Read the model definition and answer for the solid it produces. Units are mm, in the model's axes. A direction names the side the tool comes from. Round coordinates to 2 decimals unless told otherwise and drop trailing zeros. Order: outer loops, then holes, each group sorted by start corner. A loop starts at its lowest first (then second) coordinate and runs counter-clockwise, first axis right, second up. Notation, with made-up numbers: M 81.25,9 L 94.25,9 A14 ccw 94.25,24 Z; hole C -16,-12 d5. An arc over 180 degrees is marked long. Answer as CSV lines item,"result".
```python
from build123d import *

# Parameters (mm, degrees)
SALIENTE_EXTRUIR1_DEPTH = 5
REDONDEO1_R             = 30
CORTAR_EXTRUIR1_REACH   = 264.202
CROQUIS2_R              = 2


with BuildPart() as part:
    # Croquis1 → Saliente-Extruir1 (new body)
    with BuildSketch(Plane.XY):
        Polygon((-30, 0), (0, 0), (0, 5), (10, 5), (10, 215), (-150, 215), (-150, 170), (-120, 170), (-120, 175), (-40, 175), (-40, 5), (-30, 5), align=None)
    extrude(amount=SALIENTE_EXTRUIR1_DEPTH)

    # Redondeo1
    redondeo1_edges = [part.edges().sort_by_distance(p)[0] for p in [
        (-40, 175, 2.5),
        (-150, 215, 2.5),
        (10, 215, 2.5),
    ]]
    fillet(redondeo1_edges, radius=REDONDEO1_R)

    # Croquis2 → Cortar-Extruir1 (cut, up to next)
    with BuildSketch(Plane.XY.offset(5), mode=Mode.PRIVATE) as cortar_extruir1_sk1:
        with Locations((-7.5, 25)):
            Circle(CROQUIS2_R)
    cortar_extruir1_tool1 = extrude(cortar_extruir1_sk1.sketch, amount=-CORTAR_EXTRUIR1_REACH, mode=Mode.PRIVATE) & part.part
    # Croquis2 → Cortar-Extruir1 (cut, up to next)
    with BuildSketch(Plane.XY.offset(5), mode=Mode.PRIVATE) as cortar_extruir1_sk2:
        with Locations((-22.5, 25)):
            Circle(CROQUIS2_R)
    cortar_extruir1_tool2 = extrude(cortar_extruir1_sk2.sketch, amount=-CORTAR_EXTRUIR1_REACH, mode=Mode.PRIVATE) & part.part
    # Croquis2 → Cortar-Extruir1 (cut, up to next)
    with BuildSketch(Plane.XY.offset(5), mode=Mode.PRIVATE) as cortar_extruir1_sk3:
        with Locations((-127.5, 195)):
            Circle(CROQUIS2_R)
    cortar_extruir1_tool3 = extrude(cortar_extruir1_sk3.sketch, amount=-CORTAR_EXTRUIR1_REACH, mode=Mode.PRIVATE) & part.part
    # Croquis2 → Cortar-Extruir1 (cut, up to next)
    with BuildSketch(Plane.XY.offset(5), mode=Mode.PRIVATE) as cortar_extruir1_sk4:
        with Locations((-142.5, 195)):
            Circle(CROQUIS2_R)
    cortar_extruir1_tool4 = extrude(cortar_extruir1_sk4.sketch, amount=-CORTAR_EXTRUIR1_REACH, mode=Mode.PRIVATE) & part.part
    add(cortar_extruir1_tool1.solids().sort_by_distance((-7.5, 25, 5))[0], mode=Mode.SUBTRACT)
    add(cortar_extruir1_tool2.solids().sort_by_distance((-22.5, 25, 5))[0], mode=Mode.SUBTRACT)
    add(cortar_extruir1_tool3.solids().sort_by_distance((-127.5, 195, 5))[0], mode=Mode.SUBTRACT)
    add(cortar_extruir1_tool4.solids().sort_by_distance((-142.5, 195, 5))[0], mode=Mode.SUBTRACT)


solid = part.part
```
Item 1: Flat-ended cylindrical pins translate along their axes: pin 1 (2.5 mm diameter, centred on x = 3.5, z = 3.5, fed in from -Y); pin 2 (2.5 mm diameter, centred on x = -136.5, z = 3.5, fed in from -Y); pin 3 (3.5 mm diameter, centred on x = -127.5, y = 195, fed in from -Z); pin 4 (1.5 mm diameter, centred on y = 3, z = 1.5, fed in from +X). Find the tip coordinate at first contact, or state that the pin passes through.
Ans:
pin 1,"y = 5"
pin 2,"y = 170"
pin 3,"through"
pin 4,"x = 0"
Item 2: A cutting plane is placed at C-C, the plane x = -113.5. Determine the outline of the cut face in (y, z).
Ans:
outline,"M 175,0 L 215,0 L 215,5 L 175,5 Z"
Item 3: A tool of negligible diameter and unlimited length cuts with its end or side. For faces 1 (the face through (0, 2, 2)), 2 (the face through (-49.021, 166.445, 2.535)), 3 (the face through (-40, 76, 2)), from which of +Z, -Z, +X, -X, +Y, -Y can it reach the whole face along a straight path? Write none if from no direction.
Ans:
face 1,"+Z, -Z, +X, -Y"
face 2,"+Z, -Z, -Y"
face 3,"+Z, -Z, -X, -Y"
Item 4: A cutting plane is placed at A-A, the plane z = 3.7. Determine the outline of the cut face in (x, y).
Ans:
outline,"M -150,170 L -120,170 L -120,175 L -70,175 A30 cw -40,145 L -40,5 L -30,5 L -30,0 L 0,0 L 0,5 L 10,5 L 10,185 A30 ccw -20,215 L -120,215 A30 ccw -150,185 Z; hole C -142.5,195 d4; hole C -127.5,195 d4; hole C -22.5,25 d4; hole C -7.5,25 d4"
Item 5: Find the intervals of material crossed by probe 1 along X at (y, z) = (195, 1.2); probe 2 along X at (y, z) = (26.5, 2.45); probe 3 along Y at (x, z) = (-93, 0.95), in increasing order. Write a range as [from, to].
Ans:
probe 1,"[-148.28, -144.5], [-140.5, -129.5], [-125.5, 8.28]"
probe 2,"[-40, -23.82], [-21.18, -8.82], [-6.18, 10]"
probe 3,"[175, 215]"
Item 6: A cutting plane is placed at B-B, the plane y = 71.5. Determine the outline of the cut face in (x, z), and give its area (3 significant figures).
Ans:
outline,"M -40,0 L 10,0 L 10,5 L -40,5 Z"
area,"250 mm2"
Item 7: Determine the mould class of faces 4 (the face through (-120, 172, 2)), 5 (the face through (-36, 133, 0)), 6 (the face through (-95, 175, 2)), 7 (the face through (-140.979, 206.445, 2.535)) for opening direction X: +X half, -X half, draft (parallel to the pull), parting line (faces both ways), or undercut.
Ans:
face 4,"undercut"
face 5,"draft"
face 6,"undercut"
face 7,"-X half"
